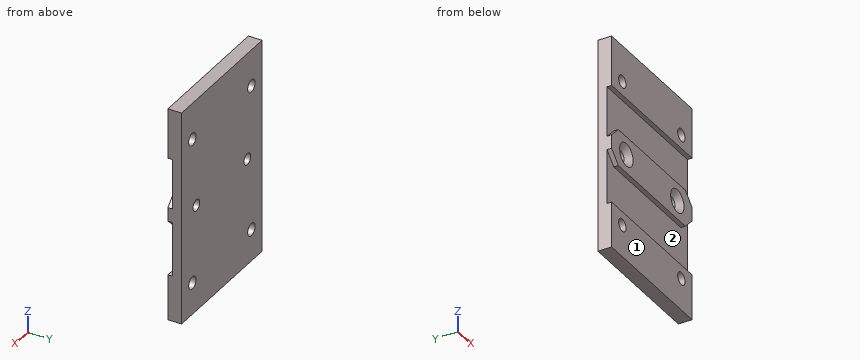
Autodesk Inventor part; units mm, degrees
ref_plane "YZ Plane" through (0, 0, 0) normal (1, 0, 0) x (0, 1, 0)
ref_plane "XZ Plane" through (0, 0, 0) normal (0, 1, 0) x (-1, 0, 0)
ref_plane "XY Plane" through (0, 0, 0) normal (0, 0, 1) x (1, 0, 0)
sketch "Esquisse1" plane through (0, 0, 0) normal (0, 1, 0) x (-1, 0, 0)
  line L0 (0, 0) -> (-60, 0)
  line L1 (-60, 0) -> (-60, 94)
  line L2 (-60, 94) -> (0, 94)
  line L3 (0, 94) -> (0, 0)
  dimension "d0" = 60
  dimension "d1" = 94
extrude "Extrusion1" add sketch "Esquisse1" along normal blind 6
sketch "Esquisse2" plane through (0, 6, 0) normal (0, 1, 0) x (1, 0, 0)
  line L0 (0, -94) -> (60, -94)
  line L1 (60, 0) -> (0, 0)
  line L2 (0, 0) -> (0, -94)
  line L3 (60, -94) -> (60, 0)
  point P0 (8, -78)
  point P1 (52, -78)
  point P2 (52, -14)
  point P3 (8, -14)
  dimension "d4" = 16
  dimension "d5" = 14
  dimension "d6" = 8
  dimension "d7" = 8
hole "Perçage1" at (8, 6, 78) at (52, 6, 78) at (52, 6, 14) at (8, 6, 14) direction (0, -1, 0) diameter 5.5 end through all
sketch "Esquisse4" plane through (0, 0, 0) normal (0, -1, 0) x (1, 0, 0)
  line L0 (0, 94) -> (0, 0)
  line L1 (60, 0) -> (60, 94)
  point P0 (11, 47)
  point P1 (49, 47)
  point P2 (0, 47)
  dimension "d15" = 11
  dimension "d16" = 11
hole "Perçage2" at (11, 0, 47) at (49, 0, 47) direction (0, 1, 0) diameter 5 end through all countersink diameter 10 countersink angle 90
sketch "Esquisse5" plane through (0, 0, 0) normal (0, -1, 0) x (1, 0, 0)
  circle A0 centre (11, 47) radius 5
  circle A1 centre (49, 47) radius 5
  circle A2 centre (52, 14) radius 2.75
  circle A3 centre (8, 78) radius 2.75
  circle A4 centre (52, 78) radius 2.75
  circle A5 centre (8, 14) radius 2.75
  line L0 (0, 0) -> (60, 0)
  line L1 (60, 0) -> (60, 94)
  line L2 (60, 94) -> (0, 94)
  line L3 (0, 94) -> (0, 0)
  line L4 (60, 0) -> (60, 94)
  line L5 (60, 72) -> (0, 72)
  line L6 (0, 72) -> (0, 55)
  line L7 (0, 55) -> (60, 55)
  line L8 (60, 55) -> (60, 72)
  line L9 (60, 39) -> (0, 39)
  line L10 (0, 39) -> (0, 20)
  line L11 (0, 20) -> (60, 20)
  line L12 (60, 20) -> (60, 39)
  dimension "d24" = 6
  dimension "d25" = 6
  dimension "d26" = 8
  dimension "d27" = 8
extrude "Extrusion2" cut sketch "Esquisse5" against normal blind 2 contours L3 L9 L1 L11 | L3 L5 L1 L7
chamfer "Chanfrein1" distance 5 angle 45 4 edges at (0, 1, 39) (0, 1, 55) (60, 1, 39) (60, 1, 55)
equation "\"d25\" = d24"
equation "\"d27\" = d26"
properties part number "attache_exterieur"
Input: part model. Units: mm. Frame: model coordinates. Face numbers are marked on the shaded views. Give positions to 0.01 mm unless a question says otherwise; leave off trailing zeros. Order: outer loops, then holes, each group sorted by start corner. A loop starts at its lowest first (then second) coordinate and runs counter-clockwise, first axis right, second up. Notation, with made-up numbers: (85.5, -30) - (102.5, -30) arc R27 ccw to (102.5, 9) - close; hole circle Ø3 at (74, -31.75). An arc over 180 degrees is marked (long way). Write each question's results on one line, items separated by ' | '.
Item 1: Section A-A (y = 1.1). Give the number of separate pieces and of enclosed holes in the cut face, and give its area (3 significant figures).
A:
separate pieces: 3 | enclosed holes: 6 | area: 3,240 mm^2
Item 2: Contact query for flat-ended pins moving along their axis: pin 1 Ø2 at (x, z) = (14, 67.5) entering from -Y; pin 2 Ø6.5 at (x, z) = (8, 14) entering from -Y. Output: stop coordinate, or through.
A:
pin 1: stops at y = 2 | pin 2: stops at y = 0
Item 3: Section B-B (z = 78). Return loops of the section in (x, y), and give its area (3 significant figures).
A:
outline: (0, 0) - (5.25, 0) - (5.25, 6) - (0, 6) - close; (10.75, 0) - (49.25, 0) - (49.25, 6) - (10.75, 6) - close; (54.75, 0) - (60, 0) - (60, 6) - (54.75, 6) - close | area: 294 mm^2
Item 4: Material intervals for line 1 along X through (y, z) = (4.4, 78); line 2 along Z through (x, y) = (19.5, 1.95); line 3 along Z through (x, y) = (54.5, 4.8), sorted ascending.
A:
line 1: x = 0 to 5.25, 10.75 to 49.25, 54.75 to 60 | line 2: z = 0 to 20, 39 to 55, 72 to 94 | line 3: z = 0 to 12.85, 15.15 to 76.85, 79.15 to 94
Item 5: Section C-C (x = 19). Return loops of the section in (y, z).
A:
outline: (0, 0) - (6, 0) - (6, 94) - (0, 94) - (0, 72) - (2, 72) - (2, 55) - (0, 55) - (0, 39) - (2, 39) - (2, 20) - (0, 20) - close
Item 6: Draft query along Z for the marked faces 1 and 2. Return one class per face: released by +Z, released by -Z, zero draft, split by the parting line, or undercut.
A:
face 1: zero draft | face 2: undercut
Item 7: Section D-D (z = 34). Return loops of the section in (x, y), and give its area (3 significant figures).
A:
outline: (0, 2) - (60, 2) - (60, 6) - (0, 6) - close | area: 240 mm^2
